```python
from build123d import *

# Parameters (mm, degrees)
F0_W     = 228.6
F0_H     = 381
F1_DEPTH = 12.7
F2_D     = 26.9875
F2_DEPTH = 25.4
F2_TIP   = 8.107862978


with BuildPart() as f1:
    # F0 (on Front) → F1 (new body)
    with BuildSketch(Plane.XZ):
        with Locations((114.3, 190.5)):
            Rectangle(F0_W, F0_H)
    extrude(amount=F1_DEPTH)

    # F2
    with Locations(Plane(origin=(0, 0, 0), x_dir=(1, 0, 0), z_dir=(0, 1, 0))):
        with Locations((177.8, -349.25), (177.8, -285.75), (177.8, -222.25), (177.8, -158.75), (177.8, -95.25), (177.8, -31.75), (50.8, -31.75), (50.8, -95.25), (50.8, -222.25), (50.8, -285.75), (50.8, -349.25), (50.8, -158.75)):
            Hole(F2_D / 2, depth=F2_DEPTH)
            with Locations((0, 0, -(F2_DEPTH + F2_TIP / 2))):  # 118° drill point
                Cone(0, F2_D / 2, F2_TIP, mode=Mode.SUBTRACT)


solid = f1.part
```
Build history of the part. All positions in model axes, mm. Coordinates: 2 decimals unless noted, no trailing zeros. Order: outer loops, then holes, each group sorted by start corner. A loop starts at its lowest first (then second) coordinate and runs counter-clockwise, first axis right, second up. Notation, with made-up numbers: (52.5, -26.75) -> (104.5, -26.75) arc R9 cw to (104.5, -20.75) -> close; hole circle Ø3 at (31, -12). An arc over 180 degrees is marked (long way). Answer in a Markdown table with one row per item. Add a question column.
Q1. Drop flat-ended pins along their axis: pin 1 (1.5 mm diameter, centred on x = 201.5, z = 313.5, fed in from +Y); pin 2 (21.5 mm diameter, centred on x = 177.8, z = 222.25, fed in from -Y). Give the stop position or say it passes through.
Q2. Band-saw the part on C-C, the plane y = -2. Give the number of separate pieces and of enclosed holes in the cut face, then the cut area to 3 significant figures.
Q3. Band-saw the part on B-B, the plane z = 95.25. List the corners of the cut face in (x, y).
Q4. Mould opens along Z. For faces 1 (the face through (43.5, -6.4, 210.9)), 2 (the face through (113, -12.7, 193)), 3 (the face through (113, -6, 381)) say: +Z half, -Z half, draft (parallel to the pull), parting line (faces both ways), or undercut.
Q5. Wall check: line 1 along X through (y, z) = (-3, 349.25); line 2 along X through (y, z) = (-8, 226.5). Give the ranges that are in metal, low to high. Write a range as [from, to].
Q6. Band-saw the part on A-A, the plane x = 177.8. List the corners of the cut face in (y, z).
Q7. Band-saw the part on D-D, the plane z = 165.5. List the corners of the cut face in (x, y).
Answers follow:
| question | item | result |
|---|---|---|
| 1 | pin 1 | y = 0 |
| 1 | pin 2 | through |
| 2 | separate pieces | 1 |
| 2 | enclosed holes | 12 |
| 2 | area | 80,200 mm^2 |
| 3 | outline | (0, -12.7) -> (37.31, -12.7) -> (37.31, 0) -> (0, 0) -> close; (64.29, -12.7) -> (164.31, -12.7) -> (164.31, 0) -> (64.29, 0) -> close; (191.29, -12.7) -> (228.6, -12.7) -> (228.6, 0) -> (191.29, 0) -> close |
| 4 | face 1 | undercut |
| 4 | face 2 | draft |
| 4 | face 3 | +Z half |
| 5 | line 1 | [0, 37.31], [64.29, 164.31], [191.29, 228.6] |
| 5 | line 2 | [0, 37.99], [63.61, 164.99], [190.61, 228.6] |
| 6 | outline | (-12.7, 0) -> (0, 0) -> (0, 18.26) -> (-12.7, 18.26) -> close; (-12.7, 45.24) -> (0, 45.24) -> (0, 81.76) -> (-12.7, 81.76) -> close; (-12.7, 108.74) -> (0, 108.74) -> (0, 145.26) -> (-12.7, 145.26) -> close; (-12.7, 172.24) -> (0, 172.24) -> (0, 208.76) -> (-12.7, 208.76) -> close; (-12.7, 235.74) -> (0, 235.74) -> (0, 272.26) -> (-12.7, 272.26) -> close; (-12.7, 299.24) -> (0, 299.24) -> (0, 335.76) -> (-12.7, 335.76) -> close; (-12.7, 362.74) -> (0, 362.74) -> (0, 381) -> (-12.7, 381) -> close |
| 7 | outline | (0, -12.7) -> (39.12, -12.7) -> (39.12, 0) -> (0, 0) -> close; (62.48, -12.7) -> (166.12, -12.7) -> (166.12, 0) -> (62.48, 0) -> close; (189.48, -12.7) -> (228.6, -12.7) -> (228.6, 0) -> (189.48, 0) -> close |
